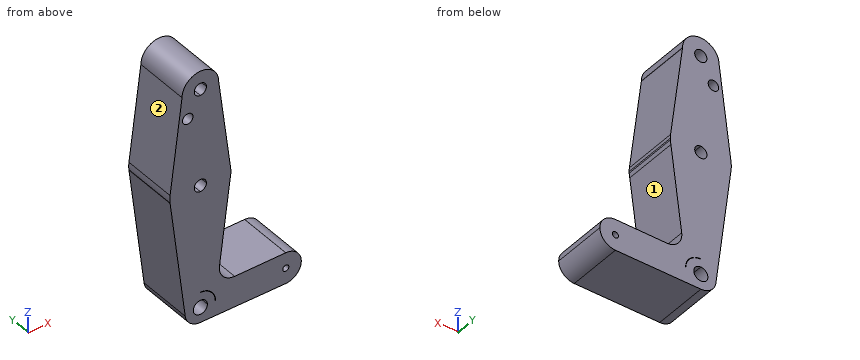
from build123d import *

# Parameters (mm, degrees)
F0_R     = 2.726595534
F1_DEPTH = 28.448


with BuildPart() as f1:
    # F0 (on Front) → F1 (new body)
    with BuildSketch(Plane.XZ):
        with BuildLine():
            ThreePointArc((-40.7547102064, 50.4481623903), (-37.9649022972, 43.7129702995), (-31.2297102064, 40.9231623903))
            ThreePointArc((-31.2297102064, 40.9231623903), (-24.5651627011, 43.6430590443), (-21.7067843213, 50.2493972355))
            ThreePointArc((-21.7067843213, 50.2493972355), (-21.7052287492, 50.3487744022), (-21.7047102064, 50.4481623903))
            ThreePointArc((-21.7047102064, 50.4481623903), (-31.2297102064, 59.9731623903), (-40.7547102064, 50.4481623903))
        make_face()
        with BuildLine():
            ThreePointArc((-28.0547102064, 50.4481623903), (-28.9846461761, 48.20309836), (-31.2297102064, 47.2731623903))
            ThreePointArc((-31.2297102064, 47.2731623903), (-33.4747742367, 52.6932264205), (-28.0547102064, 50.4481623903))
        make_face(mode=Mode.SUBTRACT)
        with BuildLine():
            ThreePointArc((-21.7067843213, 50.2493972355), (-24.5651627011, 43.6430590443), (-31.2297102064, 40.9231623903))
            Line((-31.2297102064, 40.9231623903), (-31.2297102064, 15.875))
            ThreePointArc((-31.2297102064, 15.875), (-20.7472149459, 11.9219511035), (-15.485231978, 2.0315093686))
            Line((-15.485231978, 2.0315093686), (-21.7067843213, 50.2493972355))
        make_face()
        with BuildLine():
            Line((-31.2297102064, 15.875), (-31.2297102064, 40.9231623903))
            ThreePointArc((-31.2297102064, 40.9231623903), (-37.9649022972, 43.7129702995), (-40.7547102064, 50.4481623903))
            Line((-40.7547102064, 50.4481623903), (-46.9753299172, 2.0226430538))
            ThreePointArc((-46.9753299172, 2.0226430538), (-41.7155617818, 11.918999192), (-31.2297102064, 15.875))
        make_face()
        with Locations((-37.7813987434, 37.9448458552)):
            Circle(F0_R, mode=Mode.SUBTRACT)
        with BuildLine():
            ThreePointArc((-15.485231978, 2.0315093686), (-20.7472149459, 11.9219511035), (-31.2297102064, 15.875))
            Line((-31.2297102064, 15.875), (-31.2297102064, 3.175))
            ThreePointArc((-31.2297102064, 3.175), (-28.9846461761, 2.2450640303), (-28.0547102064, 0))
            ThreePointArc((-28.0547102064, 0), (-28.9846461761, -2.2450640303), (-31.2297102064, -3.175))
            Line((-31.2297102064, -3.175), (-31.2297102064, -15.875))
            ThreePointArc((-31.2297102064, -15.875), (-21.1855906399, -12.2935465645), (-15.6734454391, -3.1651621585))
            Line((-15.6734454391, -3.1651621585), (-15.3785323056, -0.8693584745))
            ThreePointArc((-15.3785323056, -0.8693584745), (-15.3606668487, -0.4348423995), (-15.3547102064, 0))
            ThreePointArc((-15.3547102064, 0), (-15.3873742537, 1.0178489878), (-15.485231978, 2.0315093686))
        make_face()
        with BuildLine():
            Line((-31.2297102064, 3.175), (-31.2297102064, 15.875))
            ThreePointArc((-31.2297102064, 15.875), (-41.7155617818, 11.918999192), (-46.9753299172, 2.0226430538))
            ThreePointArc((-46.9753299172, 2.0226430538), (-47.1044165332, 0.0965610555), (-46.998770155, -1.8309487529))
            Line((-46.998770155, -1.8309487529), (-46.9631299673, -2.1154497456))
            ThreePointArc((-46.9631299673, -2.1154497456), (-41.6803766992, -11.9498617086), (-31.2297102064, -15.875))
            Line((-31.2297102064, -15.875), (-31.2297102064, -3.175))
            ThreePointArc((-31.2297102064, -3.175), (-34.4047102064, 0), (-31.2297102064, 3.175))
        make_face()
        with BuildLine():
            ThreePointArc((21.293102882, -63.8518376097), (18.9286306717, -58.1434967317), (13.2202897936, -55.7790245213))
            ThreePointArc((13.2202897936, -55.7790245213), (7.5119489155, -58.1434967317), (5.1474767052, -63.8518376097))
            ThreePointArc((5.1474767052, -63.8518376097), (7.5032669549, -69.5514833024), (13.1957148264, -71.9246132929))
            ThreePointArc((13.1957148264, -71.9246132929), (18.9199354863, -69.5688604485), (21.293102882, -63.8518376097))
        make_face()
        with BuildLine():
            ThreePointArc((14.8077897936, -63.8518376097), (13.2202897936, -65.4393376097), (11.6327897936, -63.8518376097))
            ThreePointArc((11.6327897936, -63.8518376097), (13.2202897936, -62.2643376097), (14.8077897936, -63.8518376097))
        make_face(mode=Mode.SUBTRACT)
        with BuildLine():
            Line((-46.9631299673, -2.1154497456), (-46.998770155, -1.8309487529))
            ThreePointArc((-46.998770155, -1.8309487529), (-46.9815923849, -1.9732797148), (-46.9631299673, -2.1154497456))
        make_face()
        with BuildLine():
            ThreePointArc((-15.6734454391, -3.1651621585), (-21.1855906399, -12.2935465645), (-31.2297102064, -15.875))
            Line((-31.2297102064, -15.875), (-31.2297102064, -55.9143376097))
            ThreePointArc((-31.2297102064, -55.9143376097), (-25.6170501307, -58.2391775341), (-23.2922102064, -63.8518376097))
            Line((-23.2922102064, -63.8518376097), (5.1474767052, -63.8518376097))
            ThreePointArc((5.1474767052, -63.8518376097), (7.5119489155, -58.1434967317), (13.2202897936, -55.7790245213))
            Line((13.2202897936, -55.7790245213), (-13.3815098989, -55.859982763))
            ThreePointArc((-13.3815098989, -55.859982763), (-19.3667419826, -53.1702109374), (-21.2911113125, -46.896880223))
            Line((-21.2911113125, -46.896880223), (-15.6734454391, -3.1651621585))
        make_face()
        with BuildLine():
            Line((-31.2297102064, -55.9143376097), (-31.2297102064, -15.875))
            ThreePointArc((-31.2297102064, -15.875), (-41.6803766992, -11.9498617086), (-46.9631299673, -2.1154497456))
            Line((-46.9631299673, -2.1154497456), (-39.1056512957, -64.8384774671))
            ThreePointArc((-39.1056512957, -64.8384774671), (-37.1809857049, -58.5995784586), (-31.2297102064, -55.9143376097))
        make_face()
        with BuildLine():
            ThreePointArc((-15.6734454391, -3.1651621585), (-15.4840904226, -2.0226424854), (-15.3785323056, -0.8693584745))
            Line((-15.3785323056, -0.8693584745), (-15.6734454391, -3.1651621585))
        make_face()
        with BuildLine():
            Line((-31.2297102064, -56.0912296504), (-31.2297102064, -55.9143376097))
            ThreePointArc((-31.2297102064, -55.9143376097), (-37.1809857049, -58.5995784586), (-39.1056512957, -64.8384774671))
            ThreePointArc((-39.1056512957, -64.8384774671), (-36.4910987194, -69.7950435766), (-31.2540792155, -71.7893002019))
            ThreePointArc((-31.2540792155, -71.7893002019), (-25.6256724995, -69.4731068285), (-23.2922102064, -63.8518376097))
            Line((-23.2922102064, -63.8518376097), (-23.469102247, -63.8518376097))
            ThreePointArc((-23.469102247, -63.8518376097), (-36.7172887206, -69.3394161239), (-31.2297102064, -56.0912296504))
        make_face()
        with BuildLine():
            Line((5.1474767052, -63.8518376097), (-23.2922102064, -63.8518376097))
            ThreePointArc((-23.2922102064, -63.8518376097), (-25.6256724995, -69.4731068285), (-31.2540792155, -71.7893002019))
            Line((-31.2540792155, -71.7893002019), (13.1957148264, -71.9246132929))
            ThreePointArc((13.1957148264, -71.9246132929), (7.5032669549, -69.5514833024), (5.1474767052, -63.8518376097))
        make_face()
        with BuildLine():
            Line((-31.2297102064, -60.1843108323), (-31.2297102064, -56.0912296504))
            ThreePointArc((-31.2297102064, -56.0912296504), (-36.7172887206, -69.3394161239), (-23.469102247, -63.8518376097))
            Line((-23.469102247, -63.8518376097), (-27.562183429, -63.8518376097))
            ThreePointArc((-27.562183429, -63.8518376097), (-33.8230432609, -66.4451706642), (-31.2297102064, -60.1843108323))
        make_face()
        with BuildLine():
            ThreePointArc((-23.469102247, -63.8518376097), (-25.7421316922, -58.3642590955), (-31.2297102064, -56.0912296504))
            Line((-31.2297102064, -56.0912296504), (-31.2297102064, -60.1843108323))
            ThreePointArc((-31.2297102064, -60.1843108323), (-28.6363771519, -61.2585045552), (-27.562183429, -63.8518376097))
            Line((-27.562183429, -63.8518376097), (-23.469102247, -63.8518376097))
        make_face()
    extrude(amount=F1_DEPTH)


solid = f1.part
Check sheet for the modelled part. Datum: model origin and axes. Units: mm. Face numbers are marked on the shaded views. A direction names the side the tool comes from. Give positions to 0.01 mm unless a question says otherwise; leave off trailing zeros. Order: outer loops, then holes, each group sorted by start corner. A loop starts at its lowest first (then second) coordinate and runs counter-clockwise, first axis right, second up. Notation, with made-up numbers: M 10.25,87 L 31.25,87 A20 cw 31.25,99 Z; hole C 22,25 d6. An arc over 180 degrees is marked long. Answer as CSV lines item,"result". Start each with the question number.
Item 1: Cross-section at B-B on x = -9. Enter the section's corners in (y, z).
Item 2: Cross-section at A-A on y = -14.5. State how many separate pieces and enclosed holes the cut face has, plus the area to 3 significant figures.
Item 3: Thickness scan on line 1 (Z direction, x = -29.5, y = -25.25); line 2 (Z direction, x = -33.5, y = -6.25); line 3 (Z direction, x = 6.5, y = -18.5). Record the ranges inside material, lowest first. Write a range as [from, to].
Item 4: Tool access check on the marked faces 1 and 2. Record the directions out of +Z, -Z, +X, -X, +Y, -Y that give a thin tool (end or side, any length) a straight path to the whole face; none if there is none.
Item 5: Gauge pin test, flat ends, axial feed: P1, Ø6, axis at x = -31.23, z = -63.85, coming from the -Y side; P2, Ø2, axis at x = 7.5, y = -25, coming from the -Z side; P3, Ø4, axis at x = -26, y = -15.5, coming from the +Z side; P4, Ø4, axis at y = -14, z = 36, coming from the -X side. Record the tip position at first contact, or that the pin passes through.
Item 6: Cross-section at C-C on z = 18. Enter the section's corners in (x, y).
Established:
1,outline,"M -28.45,-71.86 L 0,-71.86 L 0,-55.85 L -28.45,-55.85 Z"
2,separate pieces,"1"
2,enclosed holes,"6"
2,area,"3,630 mm^2"
3,line 1,"z = [-71.79, -67.09], [-60.62, -56.29], [-56.11, -2.66], [2.66, 47.79], [53.11, 59.81]"
3,line 2,"z = [-71.46, -66.73], [-60.97, -2.22], [2.22, 48.23], [52.67, 59.7]"
3,line 3,"z = [-71.9, -55.8]"
4,face 1,"+X, +Y, -Y"
4,face 2,"+Z, -X, +Y, -Y"
5,P1,"passes through"
5,P2,"stops at z = -71.91"
5,P3,"stops at z = 59.41"
5,P4,"stops at x = -42.87"
6,outline,"M -44.92,-28.45 L -17.55,-28.45 L -17.55,0 L -44.92,0 Z"
